Read the model definition and answer for the solid it produces. Units are mm, in the model's axes. Give positions to 0.01 mm unless a question says otherwise; leave off trailing zeros. Write each loop counter-clockwise with the first axis right and the second up, starting at its lowest first coordinate (ties: lowest second). Pieces come first, ordered by that corner, then holes. Notation, with made-up numbers: M 38.25,28 L 82.25,28 A26 cw 82.25,54 Z; hole C 46.5,30.5 d7. An arc over 180 degrees is marked long. Put each result on its own line as item: value.
from build123d import *

# Parameters (mm, degrees)
SKETCH1_W           = 38.06737889
SKETCH1_H           = 30.508545283
SKETCH1_R           = 1.5
SKETCH1_W_2         = 19
SKETCH1_H_2         = 19
SKETCH1_W_3         = 5.72
SKETCH1_H_3         = 4.4
BOSS_EXTRUDE1_DEPTH = 2
SKETCH2_W           = 5.72
SKETCH2_H           = 2
SKETCH2_W_2         = 19
BOSS_EXTRUDE2_DEPTH = 2
SKETCH4_W           = 5.306249276
SKETCH4_H           = 7.407734137
SKETCH4_W_2         = 4.41311821
SKETCH4_H_2         = 5.936694734
BOSS_EXTRUDE3_DEPTH = 2
SKETCH5_R           = 1.5
CUT_EXTRUDE1_DEPTH  = 10


with BuildPart() as part:
    # Sketch1 → Boss-Extrude1 (new body)
    # profile 1 of 3: a face of its own
    with BuildSketch(Plane(origin=(0, 0, 0), x_dir=(1, 0, 0), z_dir=(0, 1, 0))):
        with Locations((-9.154760873, 9.406137061)):
            Rectangle(SKETCH1_W, SKETCH1_H)
        with Locations(Location((-21.5, 7.875, 0), (0, 0, 270))):
            Circle(SKETCH1_R, mode=Mode.SUBTRACT)
        with Locations(Location((2.5, 7.875, 0), (0, 0, 270))):
            Circle(SKETCH1_R, mode=Mode.SUBTRACT)
        with Locations((-9.5, 9.5)):
            Rectangle(SKETCH1_W_2, SKETCH1_H_2, mode=Mode.SUBTRACT)
    # profile 2 of 3: a face of its own
    with BuildSketch(Plane(origin=(0, 0, 0), x_dir=(1, 0, 0), z_dir=(0, 1, 0))):
        with Locations((-16.14, 16.8)):
            Rectangle(SKETCH1_W_3, SKETCH1_H_3)
    # profile 3 of 3: a face of its own
    with BuildSketch(Plane(origin=(0, 0, 0), x_dir=(1, 0, 0), z_dir=(0, 1, 0))):
        with Locations((-2.86, 16.8)):
            Rectangle(SKETCH1_W_3, SKETCH1_H_3)
    extrude(amount=BOSS_EXTRUDE1_DEPTH)

    # Sketch2 → Boss-Extrude2 (add)
    with BuildSketch(Plane.XZ):
        with Locations((-16.14, -13.6)):
            Rectangle(SKETCH2_W, SKETCH2_H)
        with Locations((-2.86, -13.6)):
            Rectangle(SKETCH2_W, SKETCH2_H)
        with Locations((-9.5, -1)):
            Rectangle(SKETCH2_W_2, SKETCH2_H)
    extrude(amount=-BOSS_EXTRUDE2_DEPTH)

    # Sketch4 → Boss-Extrude3 (add)
    with BuildSketch(Plane(origin=(0, 2, 0), x_dir=(1, 0, 0), z_dir=(0, 1, 0))):
        with Locations((-22.157698454, 8.69688592)):
            Rectangle(SKETCH4_W, SKETCH4_H)
        with Locations((2.928777081, 8.329126069)):
            Rectangle(SKETCH4_W_2, SKETCH4_H_2)
    extrude(amount=-BOSS_EXTRUDE3_DEPTH)

    # Sketch5 → Cut-Extrude1 (cut)
    with BuildSketch(Plane(origin=(0, 2, 0), x_dir=(1, 0, 0), z_dir=(0, 1, 0))):
        with Locations(Location((-21.5, 7.3, 0), (0, 0, 270))):
            Circle(SKETCH5_R)
        with Locations(Location((2.5, 7.3, 0), (0, 0, 270))):
            Circle(SKETCH5_R)
    extrude(amount=-CUT_EXTRUDE1_DEPTH, mode=Mode.SUBTRACT)


solid = part.part
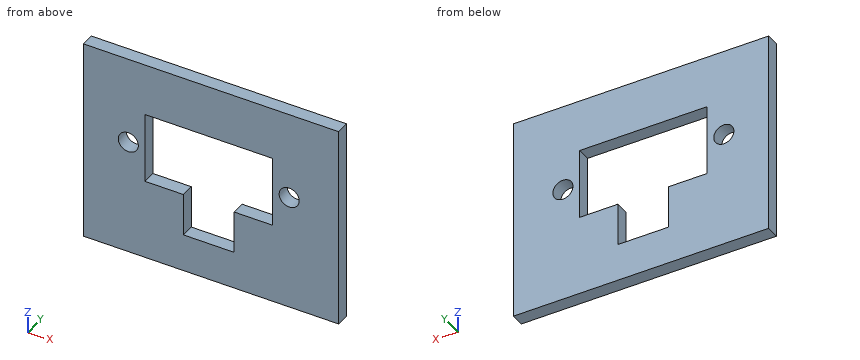
(1) Section D-D on z = -7.3 is taken. Determine the outline of the cut face in (x, y), and give its area (3 significant figures).
Result:
outline: M -28.19,0 L -23,0 L -23,2 L -28.19,2 Z; M -20,0 L -19,0 L -19,2 L -20,2 Z; M 0,0 L 1,0 L 1,2 L 0,2 Z; M 4,0 L 9.88,0 L 9.88,2 L 4,2 Z
area: 26.1 mm²
(2) Section B-B on x = -11 is taken. Determine the outline of the cut face in (y, z), and give its area (3 significant figures).
Result:
outline: M 0,-24.66 L 2,-24.66 L 2,-19 L 0,-19 Z; M 0,-2 L 2,-2 L 2,5.85 L 0,5.85 Z
area: 27.0 mm²
(3) Straight lines are drawn through the part: line 1 along X through (y, z) = (1.1, -7.3); line 2 along Z through (x, y) = (-6.5, 1.25); line 3 along Z through (x, y) = (-4.5, 1.55). For each, find the intervals that lie inside material, in ascending order. Write a range as from..to.
Result:
line 1: x = -28.19..-23, -20..-19, 0..1, 4..9.88
line 2: z = -24.66..-19, -2..5.85
line 3: z = -24.66..-12.6, -2..5.85
(4) Section A-A on z = -17 is taken. Determine the outline of the cut face in (x, y).
Result:
outline: M -28.19,0 L -13.28,0 L -13.28,2 L -28.19,2 Z; M -5.72,0 L 9.88,0 L 9.88,2 L -5.72,2 Z
(5) Section C-C on y = 0.55 is taken. Determine the outline of the cut face in (x, z).
Result:
outline: M -28.19,-24.66 L 9.88,-24.66 L 9.88,5.85 L -28.19,5.85 Z; hole C -21.5,-7.3 d3; hole M -19,-12.6 L -13.28,-12.6 L -13.28,-19 L -5.72,-19 L -5.72,-12.6 L 0,-12.6 L 0,-2 L -19,-2 Z; hole C 2.5,-7.3 d3
